Source: three-view drawing plus pictorial views. Frame: mm from the lowest corner of the part. A direction names the side the tool comes from. Give positions to 0.01 mm unless a question says otherwise; leave off trailing zeros. Loops run counter-clockwise (first coordinate to the right, second up) from the corner with the lowest first, then second, coordinate; pieces in that order, holes last. Notation, with made-up numbers: (14, 13) - (32, 13) arc R18 ccw to (32, 22) - close; hole circle Ø6 at (60, 83). An arc over 180 degrees is marked (long way). Write each question's results on one line, items separated by ' | '. Start each with the question number.
(1) Contact query for flat-ended pins moving along their axis: pin 1 (3 mm diameter, centred on x = 30, z = 6, fed in from +Y); pin 2 (8 mm diameter, centred on y = 28.5, z = 4, fed in from -X); pin 3 (1.5 mm diameter, centred on x = 21, y = 28, fed in from +Z); pin 4 (3 mm diameter, centred on y = 29, z = 5, fed in from +X). Output: stop coordinate, or through.
(2) Cut plane D-D on z = 16. Return the cut outline in (x, y).
(3) Cut plane A-A on y = 36.5. Return the cut outline in (x, z).
(4) Reachability of the marked faces 1, 2 and 3 from +Z, -Z, +X, -X, +Y, -Y: full face, straight path, thin tool, end or side. Return the list, or none.
(5) Cut plane C-C on x = 23. Return the cut outline in (y, z).
(6) Material intervals for line 1 along X through (y, z) = (16, 19.75); line 2 along X through (y, z) = (27, 4.5), sorted ascending. Write a range as [from, to].
(7) Cut plane B-B on z = 6. Return the cut outline in (x, y).
(8) Pull-direction query (Y, two-part tool) for the marked faces 4, 5 and 6; classes: pulls with the +Y half, pulls with the -Y half, needs draft (parallel to the pull), parting line crosses it, or undercut.
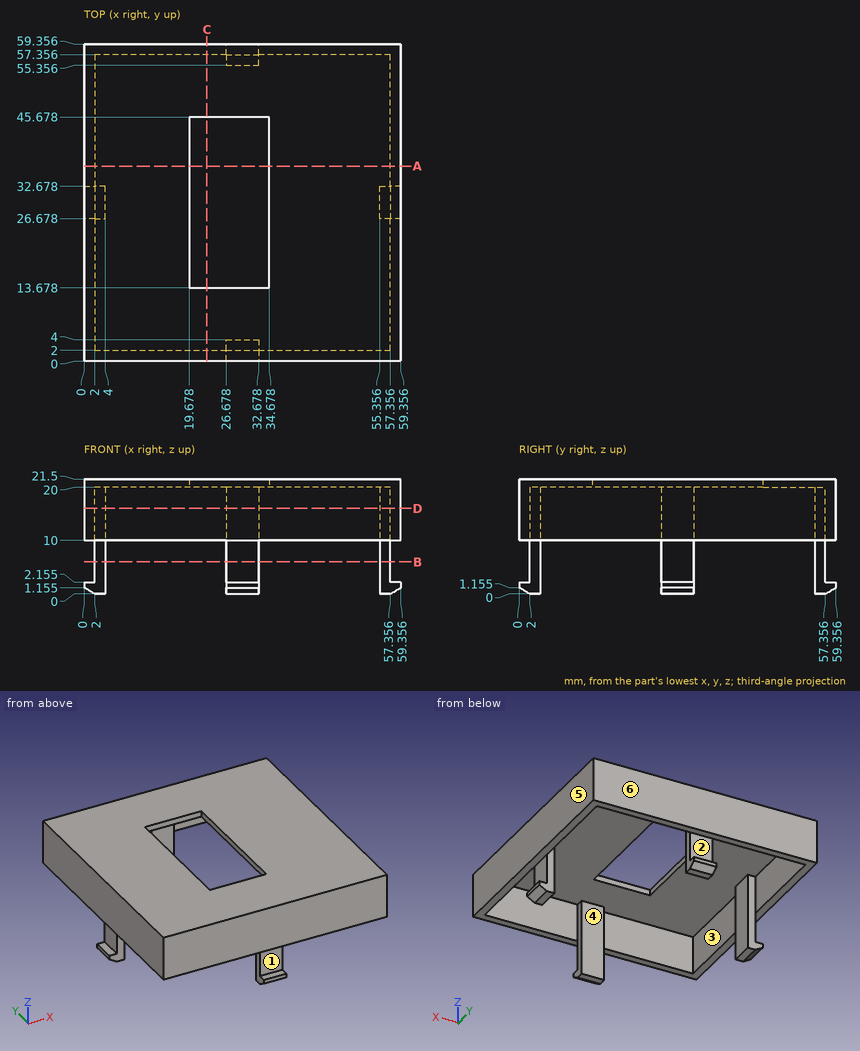
Ans:
1) pin 1: y = 57.36 | pin 2: x = 0 | pin 3: through | pin 4: x = 57.36
2) outline: (0, 0) - (59.36, 0) - (59.36, 59.36) - (0, 59.36) - close; hole (2, 2) - (26.68, 2) - (26.68, 4) - (32.68, 4) - (32.68, 2) - (57.36, 2) - (57.36, 26.68) - (55.36, 26.68) - (55.36, 32.68) - (57.36, 32.68) - (57.36, 57.36) - (32.68, 57.36) - (32.68, 55.36) - (26.68, 55.36) - (26.68, 57.36) - (2, 57.36) - (2, 32.68) - (4, 32.68) - (4, 26.68) - (2, 26.68) - close
3) outline: (0, 10) - (2, 10) - (2, 20) - (19.68, 20) - (19.68, 21.5) - (0, 21.5) - close; (34.68, 20) - (57.36, 20) - (57.36, 10) - (59.36, 10) - (59.36, 21.5) - (34.68, 21.5) - close
4) face 1: +X, -X, -Y | face 2: +X, -X, +Y | face 3: -Z
5) outline: (0, 10) - (2, 10) - (2, 20) - (13.68, 20) - (13.68, 21.5) - (0, 21.5) - close; (45.68, 20) - (57.36, 20) - (57.36, 10) - (59.36, 10) - (59.36, 21.5) - (45.68, 21.5) - close
6) line 1: [0, 2], [57.36, 59.36] | line 2: [2, 4], [55.36, 57.36]
7) outline: (2, 26.68) - (4, 26.68) - (4, 32.68) - (2, 32.68) - close; (26.68, 2) - (32.68, 2) - (32.68, 4) - (26.68, 4) - close; (26.68, 55.36) - (32.68, 55.36) - (32.68, 57.36) - (26.68, 57.36) - close; (55.36, 26.68) - (57.36, 26.68) - (57.36, 32.68) - (55.36, 32.68) - close
8) face 4: undercut | face 5: needs draft | face 6: pulls with the +Y half
